Design review of the part built by this model. Coordinates are the model's own, in mm. Face numbers are marked on the shaded views. Give positions to 0.01 mm unless a question says otherwise; leave off trailing zeros. Loops run counter-clockwise (first coordinate to the right, second up) from the corner with the lowest first, then second, coordinate; pieces in that order, holes last. Notation, with made-up numbers: M -30,2.25 L -18,2.25 A28 ccw -18,34.25 Z; hole C 58.5,87.5 d2. An arc over 180 degrees is marked long. Use a Markdown table: item, result. Add a question column.
(1) Add section A-A, the plane z = 0. Give the boundary of the cut face in (x, y), then the cut area to 3 significant figures.
(2) Draft analysis for pull direction Z (two halves, no side actions). For the marked faces 1, 2 and 3, state which applies: pulls with the +Z half, pulls with the -Z half, needs draft (parallel to the pull), parting line crosses it, or undercut.
(3) For probe 1 along Z at (x, y) = (0, -2.25); probe 2 along X at (y, z) = (7.5, -7.5); probe 3 along X at (y, z) = (-2.5, 7), list the stretches that pass through material, from the lowest coordinate up.
(4) Insertion check: pin 1 Ø1.5 at (x, z) = (11.5, 1.5) entering from +Y. The pin has a flat end and moves straight along its axis. Give the tip position at first contact, or say it passes through.
(5) Add section D-D, the plane z = 17.5. Give the boundary of the cut face in (x, y).
(6) Add section C-C, the plane y = -5. Give the boundary of the cut face in (x, z).
(7) Add section B-B, the plane x = 0. Give the boundary of the cut face in (y, z).
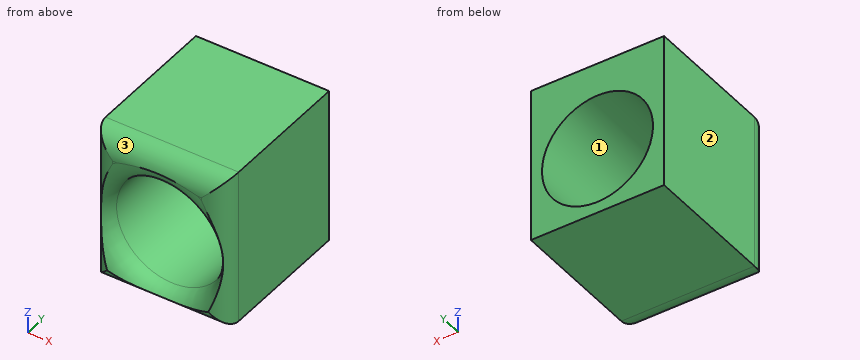
```python
from build123d import *

# Parameters (mm, degrees)
F0_W        = 30
F0_H        = 30
F0_R        = 12.5
F1_DEPTH    = 17.5
F2_DEPTH    = 5
F3_T1_DEPTH = 55
F3_T3_DEPTH = 60


# Not quite as in the source:
# - a fillet or chamfer that OpenCascade refuses, or shapes differently, is made with other operations: its cross-section is extruded or revolved along the edge and cut away or added


with BuildPart() as f1:
    # F0 (on Front) → F1 (new body, symmetric)
    with BuildSketch(Plane.XZ):
        Rectangle(F0_W, F0_H)
        Circle(F0_R, mode=Mode.SUBTRACT)
    extrude(amount=F1_DEPTH, both=True)

    # F2 (add): a face of the model
    f2_faces = [f1.faces().sort_by_distance(p)[0] for p in [
        (0, 0, 15),
    ]]
    extrude(f2_faces, amount=F2_DEPTH)

    # F3: fillet of radius 5 on 5 edges, made by hand

    # F3_s2 → F3_t1 (cut)
    with BuildSketch(Plane.YZ.offset(-27.5)):
        with BuildLine():
            ThreePointArc((-12.5, -15), (-16.0355339059, -13.5355339059), (-17.5, -10))
            Line((-17.5, -10), (-17.5, -15))
            Line((-17.5, -15), (-12.5, -15))
        make_face()
        with BuildLine():
            ThreePointArc((-17.5, 15), (-16.0355339059, 18.5355339059), (-12.5, 20))
            Line((-12.5, 20), (-17.5, 20))
            Line((-17.5, 20), (-17.5, 15))
        make_face()
    extrude(amount=F3_T1_DEPTH, mode=Mode.SUBTRACT)

    # F3_s4 → F3_t3 (cut)
    with BuildSketch(Plane.XY.offset(-27.5)):
        with BuildLine():
            ThreePointArc((15, -12.5), (13.5355339059, -16.0355339059), (10, -17.5))
            Line((10, -17.5), (15, -17.5))
            Line((15, -17.5), (15, -12.5))
        make_face()
        with BuildLine():
            ThreePointArc((-15, -12.5), (-13.5355339059, -16.0355339059), (-10, -17.5))
            Line((-10, -17.5), (-15, -17.5))
            Line((-15, -17.5), (-15, -12.5))
        make_face()
    extrude(amount=F3_T3_DEPTH, mode=Mode.SUBTRACT)

    # F3_s5 → F3_t6 (revolve, cut)
    with BuildSketch(Plane.XY):
        with BuildLine():
            ThreePointArc((17.5, -17.5), (13.9644660941, -16.0355339059), (12.5, -12.5))
            Line((12.5, -12.5), (12.5, -17.5))
            Line((12.5, -17.5), (17.5, -17.5))
        make_face()
    revolve(axis=Axis((0, -17.5, 0), (0, -1, 0)), mode=Mode.SUBTRACT)


solid = f1.part
```
Established:
| question | item | result |
|---|---|---|
| 1 | outline | M -15,-12.5 A5 ccw -13.75,-15.81 A5 ccw -12.5,-12.5 L -12.5,17.5 L -15,17.5 Z; M 12.5,-12.5 A5 ccw 13.75,-15.81 A5 ccw 15,-12.5 L 15,17.5 L 12.5,17.5 Z |
| 1 | area | 161 mm^2 |
| 2 | face 1 | undercut |
| 2 | face 2 | needs draft |
| 2 | face 3 | pulls with the +Z half |
| 3 | probe 1 | -15 to -12.5, 12.5 to 20 |
| 3 | probe 2 | -15 to -10, 10 to 15 |
| 3 | probe 3 | -15 to -10.36, 10.36 to 15 |
| 4 | pin 1 | through |
| 5 | outline | M -15,-12.5 A5 ccw -12.5,-16.83 L 12.5,-16.83 A5 ccw 15,-12.5 L 15,17.5 L -15,17.5 Z |
| 6 | outline | M -15,-15 L 15,-15 L 15,20 L -15,20 Z; hole C 0,0 d25 |
| 7 | outline | M -17.34,16.25 A5 ccw -12.5,12.5 L 17.5,12.5 L 17.5,20 L -12.5,20 A5 ccw Z; M -15.81,-13.75 A5 ccw -12.5,-15 L 17.5,-15 L 17.5,-12.5 L -12.5,-12.5 A5 ccw Z |
